Could you check a few things on this model? Use its own coordinates, in mm. Face numbers are marked on the shaded views. Give positions to 0.01 mm unless a question says otherwise; leave off trailing zeros. Order: outer loops, then holes, each group sorted by start corner. A loop starts at its lowest first (then second) coordinate and runs counter-clockwise, first axis right, second up. Notation, with made-up numbers: M -2.5,14 L 21.5,14 A25 cw 21.5,39 Z; hole C 16,6.5 d6. An arc over 180 degrees is marked long. Use a Markdown table: item, result. Add a question column.
```python
from build123d import *

# Parameters (mm, degrees)
EXTRUDE_1_DEPTH     = 3
EXTRUDE_2_DEPTH     = 6
SKETCH_3_R          = 2.2
CUT_EXTRUDE_1_DEPTH = 188.979387168


with BuildPart() as part:
    # 草图1 → 凸台-拉伸1 (new body)
    with BuildSketch(Plane(origin=(0, 0, 0), x_dir=(1, 0, 0), z_dir=(0, 1, 0))):
        with BuildLine():
            Line((10, 0), (117.5, 0))
            ThreePointArc((117.5, 0), (124.571067812, 2.928932188), (127.5, 10))
            Line((127.5, 10), (127.5, 128))
            ThreePointArc((127.5, 128), (124.571067812, 135.071067812), (117.5, 138))
            Line((117.5, 138), (10, 138))
            ThreePointArc((10, 138), (2.928932188, 135.071067812), (0, 128))
            Line((0, 128), (0, 10))
            ThreePointArc((0, 10), (2.928932188, 2.928932188), (10, 0))
        make_face()
    extrude(amount=EXTRUDE_1_DEPTH)

    # 草图2 → 凸台-拉伸2 (add)
    with BuildSketch(Plane(origin=(0, 3, 0), x_dir=(1, 0, 0), z_dir=(0, 1, 0))):
        with BuildLine():
            Line((0, 128), (0, 10))
            ThreePointArc((0, 10), (2.928932188, 2.928932188), (10, 0))
            Line((10, 0), (117.5, 0))
            ThreePointArc((117.5, 0), (124.571067812, 2.928932188), (127.5, 10))
            Line((127.5, 10), (127.5, 128))
            ThreePointArc((127.5, 128), (124.571067812, 135.071067812), (117.5, 138))
            Line((117.5, 138), (10, 138))
            ThreePointArc((10, 138), (2.928932188, 135.071067812), (0, 128))
        make_face()
        with BuildLine():
            Line((117.5, 135), (10, 135))
            ThreePointArc((10, 135), (5.050252532, 132.949747468), (3, 128))
            Line((3, 128), (3, 10))
            ThreePointArc((3, 10), (5.050252532, 5.050252532), (10, 3))
            Line((10, 3), (117.5, 3))
            ThreePointArc((117.5, 3), (122.449747468, 5.050252532), (124.5, 10))
            Line((124.5, 10), (124.5, 128))
            ThreePointArc((124.5, 128), (122.449747468, 132.949747468), (117.5, 135))
        make_face(mode=Mode.SUBTRACT)
    extrude(amount=EXTRUDE_2_DEPTH)

    # 草图3 → 切除-拉伸1 (cut, through all)
    with BuildSketch(Plane(origin=(0, 3, 0), x_dir=(1, 0, 0), z_dir=(0, 1, 0))):
        with Locations(Location((10, 128, 0), (0, 0, 270))):
            Circle(SKETCH_3_R)
        with Locations(Location((117.5, 128, 0), (0, 0, 270))):
            Circle(SKETCH_3_R)
        with Locations(Location((10, 10, 0), (0, 0, 270))):
            Circle(SKETCH_3_R)
        with Locations(Location((117.5, 10, 0), (0, 0, 270))):
            Circle(SKETCH_3_R)
    extrude(amount=-CUT_EXTRUDE_1_DEPTH, mode=Mode.SUBTRACT)


solid = part.part
```
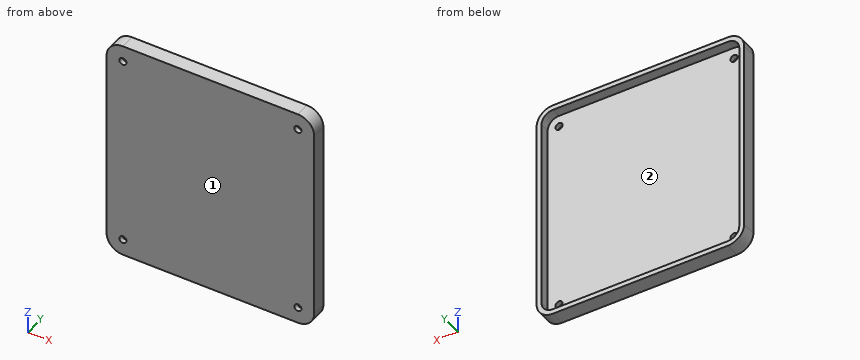
1) Please list where these lines run through material, in increasing order: line 1 (X direction, y = 8, z = -106); line 2 (Z direction, x = 117, y = 3.75); line 3 (X direction, y = 1.35, z = -10). Write a range as from..to.
2) For pin 1 (10 mm diameter, centred on x = 107.5, z = -14.5, fed in from +Y); pin 2 (4 mm diameter, centred on x = 117.5, z = -128, fed in from +Y), each with a flat end and sliding along its axis, tell me the tip position at first contact or that it passes through.
3) Suppose I cut it at A-A on y = 7. Please give me the cut outline in (x, z).
4) Suppose I cut it at C-C on z = -68. Please give me the cut outline in (x, y), and give its area (4 significant figures).
5) We'd pull the mould along X, two halves only. Please class the marked faces 1 and 2: pulls with the +X half, pulls with the -X half, needs draft (parallel to the pull), parting line crosses it, or undercut.
6) Suppose I cut it at B-B on x = 102. Please give me the cut outline in (y, z).
Values found:
| question | item | result |
|---|---|---|
| 1 | line 1 | x = 0..3, 124.5..127.5 |
| 1 | line 2 | z = -138..-135, -3..0 |
| 1 | line 3 | x = 0..7.8, 12.2..115.3, 119.7..127.5 |
| 2 | pin 1 | stops at y = 3 |
| 2 | pin 2 | passes through |
| 3 | outline | M 0,-128 A10 ccw 10,-138 L 117.5,-138 A10 ccw 127.5,-128 L 127.5,-10 A10 ccw 117.5,0 L 10,0 A10 ccw 0,-10 Z; hole M 3,-128 A7 ccw 10,-135 L 117.5,-135 A7 ccw 124.5,-128 L 124.5,-10 A7 ccw 117.5,-3 L 10,-3 A7 ccw 3,-10 Z |
| 4 | outline | M 0,0 L 127.5,0 L 127.5,9 L 124.5,9 L 124.5,3 L 3,3 L 3,9 L 0,9 Z |
| 4 | area | 418.5 mm^2 |
| 5 | face 1 | needs draft |
| 5 | face 2 | undercut |
| 6 | outline | M 0,-138 L 9,-138 L 9,-135 L 3,-135 L 3,-3 L 9,-3 L 9,0 L 0,0 Z |
